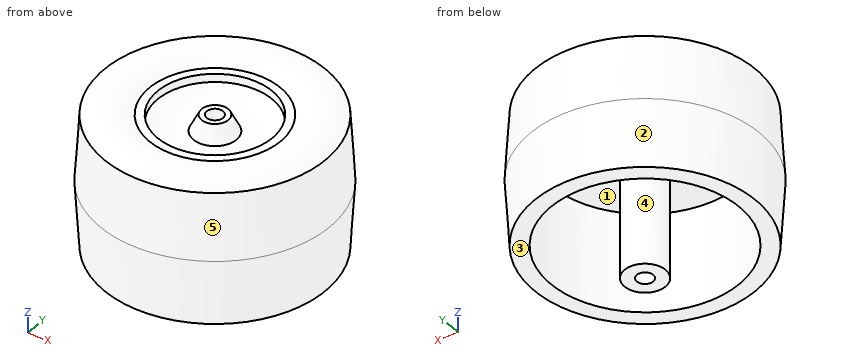
Autodesk Inventor part; units mm, degrees
ref_plane "YZ Plane" through (0, 0, 0) normal (1, 0, 0) x (0, 1, 0)
ref_plane "XZ Plane" through (0, 0, 0) normal (0, 1, 0) x (-1, 0, 0)
ref_plane "XY Plane" through (0, 0, 0) normal (0, 0, 1) x (1, 0, 0)
sketch "Sketch1" plane through (0, 0, 0) normal (1, 0, 0) x (0, 1, 0)
  line L0 (1.5875, -19.05) -> (1.5875, 12.7)
  line L1 (1.5875, 12.7) -> (2.5875, 12.7)
  line L2 (2.5875, 12.7) -> (4.175, 9.525)
  arc A0 (4.175, 9.525) -> (11.1125, 11.1125) centre (5.6612, 18.9827) ccw
  line L3 (11.1125, 11.1125) -> (11.1125, 12.7)
  line L4 (11.1125, 12.7) -> (12.7, 12.7)
  line L5 (21.4312, 12.7) -> (22.225, 0)
  line L6 (18.2563, -12.7) -> (18.2562, 6.35)
  line L7 (18.2562, 6.35) -> (3.9688, 6.35)
  line L8 (3.9688, 6.35) -> (3.9688, -19.05)
  line L9 (3.9688, -19.05) -> (1.5875, -19.05)
  arc A1 (21.4312, 12.7) -> (12.7, 12.7) centre (17.0656, 7.236) ccw
  line L10 (22.225, 0) -> (21.4312, -12.7)
  line L11 (21.4312, -12.7) -> (18.2563, -12.7)
  line L12 (0, -26.6565) -> (0, 26.5892)
  point P0 (0, 0)
  dimension "d0" = 1.5875
  dimension "d1" = 1
  dimension "d2" = 3.175
  dimension "d3" = 1.5875
  dimension "d4" = 11.1125
  dimension "d5" = 12.7
  dimension "d6" = 1.5875
  dimension "d7" = 21.4312
  dimension "d8" = 22.225
  dimension "d9" = 12.7
  dimension "d10" = 12.7
  dimension "d11" = 0
  dimension "d13" = 12.7
  dimension "d14" = 21.4312
  dimension "d15" = 3.175
  dimension "d16" = 19.05
  dimension "d17" = 2.3813
  dimension "d18" = 6.35
  dimension "d19" = 6.35
  dimension "d20" = 12.7
  dimension "d21" = 9.5738
  dimension "d22" = 6.9938
revolve "Revolution1" add sketch "Sketch1" angle 360 about axis through (0, 0, -10) along (0, 0, 1)
properties part number "launcher_wheel"
Could you check a few things on this model? Use its own coordinates, in mm. Face numbers are marked on the shaded views. A direction names the side the tool comes from. Give positions to 0.01 mm unless a question says otherwise; leave off trailing zeros. Order: outer loops, then holes, each group sorted by start corner. A loop starts at its lowest first (then second) coordinate and runs counter-clockwise, first axis right, second up.
1. Suppose I cut it at A-A (z = -11). List the corners of the cut face in (x, y) for me (1 decimal), plus the area to 3 significant figures.
2. Will these pins go through, and if not, where does the flat tip stop? P1, Ø1.6, axis at x = 1, y = 0, coming from the +Z side; P2, Ø12, axis at y = 6.5, z = 9.5, coming from the -X side; P3, Ø10, axis at x = 7, z = -13.5, coming from the -Y side; P4, Ø2.5, axis at x = 0, y = 0, coming from the -Z side.
3. We'd pull the mould along X, two halves only. Please class the marked faces 1, 2 and 3: pulls with the +X half, pulls with the -X half, needs draft (parallel to the pull), parting line crosses it, or undercut.
4. Suppose I cut it at B-B (z = 7). List the corners of the cut face in (x, y) for me (1 decimal), plus the area to 3 significant figures.
5. For the marked faces 4 and 5, which set-ups out of +Z, -Z, +X, -X, +Y, -Y let a thin tool reach every point of the face, with its end or its side?
6. I need wall thicknesses on L1, parallel to X at y = 0, z = 11.7; L2, parallel to X at y = -0.5, z = -10; L3, parallel to X at y = -3, z = 1.5. Which ranges of each line are inside material? Lowest first, please.
7. Suppose I cut it at C-C (z = -4.5). List the corners of the cut face in (x, y) for me (1 decimal).
Solved:
1. outline: circle Ø43.1 at (0, 0); circle Ø7.9 at (0, 0); hole circle Ø36.5 at (0, 0); hole circle Ø3.2 at (0, 0)
1. area: 452 mm2
2. P1: stops at z = 12.7
2. P2: stops at x = -21.79
2. P3: stops at y = -21.37
2. P4: passes through
3. face 1: undercut
3. face 2: parting line crosses it
3. face 3: needs draft
4. outline: circle Ø43.6 at (0, 0); hole circle Ø3.2 at (0, 0)
4. area: 1,480 mm2
5. face 4: -Z
5. face 5: +Z
6. L1: x = -21.49 to -11.11, -3.09 to -1.59, 1.59 to 3.09, 11.11 to 21.49
6. L2: x = -21.59 to -18.25, -3.94 to -1.51, 1.51 to 3.94, 18.25 to 21.59
6. L3: x = -21.93 to -18.01, -2.6 to 2.6, 18.01 to 21.93
7. outline: circle Ø43.9 at (0, 0); circle Ø7.9 at (0, 0); hole circle Ø36.5 at (0, 0); hole circle Ø3.2 at (0, 0)
